Source: CAD feature listing. Evaluate the final solid. Frame: model axes, mm. Face numbers are marked on the shaded views. Give positions to 0.01 mm unless a question says otherwise; leave off trailing zeros. Write each loop counter-clockwise with the first axis right and the second up, starting at its lowest first coordinate (ties: lowest second). Pieces come first, ordered by that corner, then holes. Notation, with made-up numbers: M 79,55.5 L 134,55.5 A15 ccw 134,72.5 Z; hole C -26.75,-7.75 d8. An arc over 180 degrees is marked long. Use CSV: the item, a comma, the result in double quotes. Start each with the question number.
from build123d import *

# Parameters (mm, degrees)
SKETCH1_R           = 37.500000057
BOSS_EXTRUDE1_DEPTH = 507.84
SKETCH3_R           = 35
CUT_EXTRUDE1_DEPTH  = 507.84


with BuildPart() as part:
    # Sketch1 → Boss-Extrude1 (new body)
    with BuildSketch(Plane.XY):
        Circle(SKETCH1_R)
    extrude(amount=BOSS_EXTRUDE1_DEPTH)

    # Sketch3 → Cut-Extrude1 (cut)
    with BuildSketch(Plane(origin=(0, 0, 0), x_dir=(-1, 0, 0), z_dir=(0, 0, -1))):
        Circle(SKETCH3_R)
    extrude(amount=-CUT_EXTRUDE1_DEPTH, mode=Mode.SUBTRACT)

    # Sketch9 → Groove for ANSI B27.7 - 3BM1-68_ Basic I (revolve, cut)
    with BuildSketch(Plane(origin=(0, 0, 507.84), x_dir=(0, 1, 0), z_dir=(-1, 0, 0))):
        with BuildLine():
            Line((35.7, 503.96), (31.5, 503.96))
            Line((31.5, 503.96), (31.5, 506.57))
            Line((31.5, 506.57), (35.7, 506.57))
            ThreePointArc((35.7, 506.57), (35.982842712, 506.452842712), (36.1, 506.17))
            Line((36.1, 506.17), (36.1, 504.36))
            ThreePointArc((36.1, 504.36), (35.982842712, 504.077157288), (35.7, 503.96))
        make_face()
    revolve(axis=Axis((0, 0, 557.84), (0, 0, -1)), mode=Mode.SUBTRACT)

    # Sketch11 → Groove for ANSI B27.7 - 3BM1-68_ Bas 2 (revolve, cut)
    with BuildSketch(Plane(origin=(0, 0, 507.84), x_dir=(0, 1, 0), z_dir=(-1, 0, 0))):
        with BuildLine():
            Line((35.7, 1.27), (31.5, 1.27))
            Line((31.5, 1.27), (31.5, 3.88))
            Line((31.5, 3.88), (35.7, 3.88))
            ThreePointArc((35.7, 3.88), (35.982842712, 3.762842712), (36.1, 3.48))
            Line((36.1, 3.48), (36.1, 1.67))
            ThreePointArc((36.1, 1.67), (35.982842712, 1.387157288), (35.7, 1.27))
        make_face()
    revolve(axis=Axis((0, 0, 557.84), (0, 0, -1)), mode=Mode.SUBTRACT)


solid = part.part
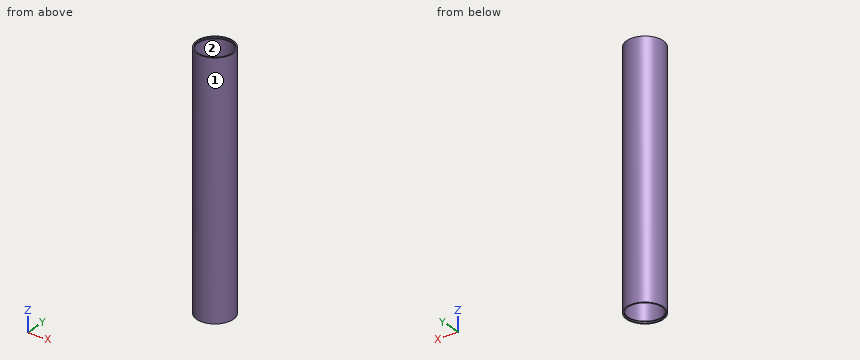
1. Line query: probe 1 along Z at (x, y) = (-19.5, -29.5); probe 2 along Y at (x, z) = (0, 507); probe 3 along Y at (x, z) = (10, 405). Output: solid intervals per line, ascending.
2. First-contact query: pin 1 (8 mm diameter, centred on y = 28, z = 104, fed in from +X); pin 2 (2 mm diameter, centred on x = -10.5, z = 305, fed in from -Y); pin 3 (12 mm diameter, centred on x = -27, z = 136, fed in from -Y). Flat tips, straight axial feed; report the tip coordinate or a pass-through.
3. Section C-C on z = 397. Return loops of the section in (x, y), then the cut area to 3 significant figures.
4. Pull-direction query (X, two-part tool) for the marked faces 1 and 2; classes: released by +X, released by -X, zero draft, split by the parting line, or undercut.
Resolved:
1,probe 1,"z = 0 to 1.27, 3.88 to 503.96, 506.57 to 507.84"
1,probe 2,"y = -37.5 to -35, 35 to 37.5"
1,probe 3,"y = -36.14 to -33.54, 33.54 to 36.14"
2,pin 1,"stops at x = 28.81"
2,pin 2,"stops at y = -36.28"
2,pin 3,"stops at y = -31.07"
3,outline,"C 0,0 d75; hole C 0,0 d70"
3,area,"569 mm2"
4,face 1,"split by the parting line"
4,face 2,"undercut"
